Part model, mm, in its own coordinate system. Round coordinates to 2 decimals unless told otherwise and drop trailing zeros. Order: outer loops, then holes, each group sorted by start corner. A loop starts at its lowest first (then second) coordinate and runs counter-clockwise, first axis right, second up. Notation, with made-up numbers: (41, 45.5) -> (96, 45.5) arc R21 cw to (96, 58.5) -> close; hole circle Ø2 at (-27, 53). An arc over 180 degrees is marked (long way). Answer as a JSON object with one key per item and string values. Group by question number.
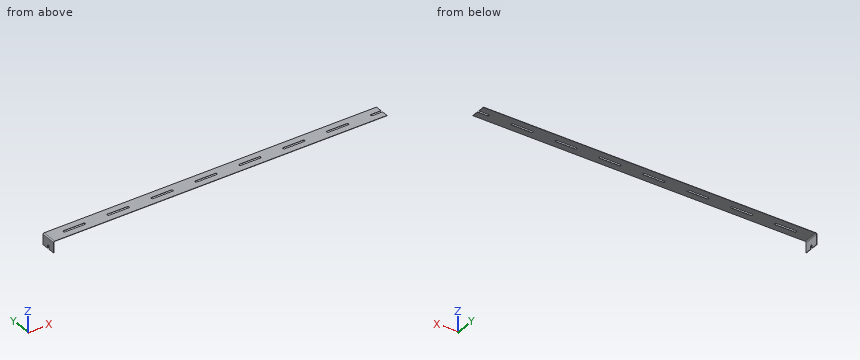
```python
from build123d import *

# Parameters (mm, degrees)
F0_W     = 3
F0_H     = 3
F1_DEPTH = 0.15
F2_DEPTH = 1.9
F3_W     = 0.15
F3_H     = 7
F4_DEPTH = 5
F6_DEPTH = 25
F7_R     = 0.5


with BuildPart() as f1:
    # F0 (on Top) → F1 (new body)
    with BuildSketch(Plane.XY):
        with Locations((72.2, 2)):
            Rectangle(F0_W, F0_H)
        with BuildLine():
            Line((10.1, -0.5), (10.1, -3.5))
            Line((10.1, -3.5), (20.2, -3.5))
            Line((20.2, -3.5), (30.3, -3.5))
            Line((30.3, -3.5), (30.3, -0.5))
            Line((30.3, -0.5), (25.7, -0.5))
            ThreePointArc((25.7, -0.5), (25.4171572875, -0.3828427125), (25.3, -0.1))
            Line((25.3, -0.1), (25.3, 0.1))
            ThreePointArc((25.3, 0.1), (25.4171572875, 0.3828427125), (25.7, 0.5))
            Line((25.7, 0.5), (30.3, 0.5))
            Line((30.3, 0.5), (30.3, 3.5))
            Line((30.3, 3.5), (20.2, 3.5))
            Line((20.2, 3.5), (10.1, 3.5))
            Line((10.1, 3.5), (10.1, 0.5))
            Line((10.1, 0.5), (14.7, 0.5))
            ThreePointArc((14.7, 0.5), (14.9828427125, 0.3828427125), (15.1, 0.1))
            Line((15.1, 0.1), (15.1, -0.1))
            ThreePointArc((15.1, -0.1), (14.9828427125, -0.3828427125), (14.7, -0.5))
            Line((14.7, -0.5), (10.1, -0.5))
        make_face()
        with BuildLine():
            Line((30.3, -0.5), (30.3, -3.5))
            Line((30.3, -3.5), (40.4, -3.5))
            Line((40.4, -3.5), (50.5, -3.5))
            Line((50.5, -3.5), (50.5, -0.5))
            Line((50.5, -0.5), (45.9, -0.5))
            ThreePointArc((45.9, -0.5), (45.6171572875, -0.3828427125), (45.5, -0.1))
            Line((45.5, -0.1), (45.5, 0.1))
            ThreePointArc((45.5, 0.1), (45.6171572875, 0.3828427125), (45.9, 0.5))
            Line((45.9, 0.5), (50.5, 0.5))
            Line((50.5, 0.5), (50.5, 3.5))
            Line((50.5, 3.5), (40.4, 3.5))
            Line((40.4, 3.5), (30.3, 3.5))
            Line((30.3, 3.5), (30.3, 0.5))
            Line((30.3, 0.5), (34.9, 0.5))
            ThreePointArc((34.9, 0.5), (35.1828427125, 0.3828427125), (35.3, 0.1))
            Line((35.3, 0.1), (35.3, -0.1))
            ThreePointArc((35.3, -0.1), (35.1828427125, -0.3828427125), (34.9, -0.5))
            Line((34.9, -0.5), (30.3, -0.5))
        make_face()
        with BuildLine():
            Line((50.5, -0.5), (50.5, -3.5))
            Line((50.5, -3.5), (60.6, -3.5))
            Line((60.6, -3.5), (70.7, -3.5))
            Line((70.7, -3.5), (70.7, -0.5))
            Line((70.7, -0.5), (66.1, -0.5))
            ThreePointArc((66.1, -0.5), (65.8171572875, -0.3828427125), (65.7, -0.1))
            Line((65.7, -0.1), (65.7, 0.1))
            ThreePointArc((65.7, 0.1), (65.8171572875, 0.3828427125), (66.1, 0.5))
            Line((66.1, 0.5), (70.7, 0.5))
            Line((70.7, 0.5), (70.7, 3.5))
            Line((70.7, 3.5), (60.6, 3.5))
            Line((60.6, 3.5), (50.5, 3.5))
            Line((50.5, 3.5), (50.5, 0.5))
            Line((50.5, 0.5), (55.1, 0.5))
            ThreePointArc((55.1, 0.5), (55.3828427125, 0.3828427125), (55.5, 0.1))
            Line((55.5, 0.1), (55.5, -0.1))
            ThreePointArc((55.5, -0.1), (55.3828427125, -0.3828427125), (55.1, -0.5))
            Line((55.1, -0.5), (50.5, -0.5))
        make_face()
        with BuildLine():
            Line((0, 3.5), (0, -3.5))
            Line((0, -3.5), (10.1, -3.5))
            Line((10.1, -3.5), (10.1, -0.5))
            Line((10.1, -0.5), (5.5, -0.5))
            ThreePointArc((5.5, -0.5), (5.2171572875, -0.3828427125), (5.1, -0.1))
            Line((5.1, -0.1), (5.1, 0.1))
            ThreePointArc((5.1, 0.1), (5.2171572875, 0.3828427125), (5.5, 0.5))
            Line((5.5, 0.5), (10.1, 0.5))
            Line((10.1, 0.5), (10.1, 3.5))
            Line((10.1, 3.5), (0, 3.5))
        make_face()
        with Locations((72.2, -2)):
            Rectangle(F0_W, F0_H)
        with BuildLine():
            Line((73.7, -0.5), (73.7, -3.5))
            Line((73.7, -3.5), (80.8, -3.5))
            Line((80.8, -3.5), (90.9, -3.5))
            Line((90.9, -3.5), (90.9, -0.5))
            Line((90.9, -0.5), (86.3, -0.5))
            ThreePointArc((86.3, -0.5), (86.0171572875, -0.3828427125), (85.9, -0.1))
            Line((85.9, -0.1), (85.9, 0.1))
            ThreePointArc((85.9, 0.1), (86.0171572875, 0.3828427125), (86.3, 0.5))
            Line((86.3, 0.5), (90.9, 0.5))
            Line((90.9, 0.5), (90.9, 3.5))
            Line((90.9, 3.5), (80.8, 3.5))
            Line((80.8, 3.5), (73.7, 3.5))
            Line((73.7, 3.5), (73.7, 0.5))
            Line((73.7, 0.5), (75.3, 0.5))
            ThreePointArc((75.3, 0.5), (75.5828427125, 0.3828427125), (75.7, 0.1))
            Line((75.7, 0.1), (75.7, -0.1))
            ThreePointArc((75.7, -0.1), (75.5828427125, -0.3828427125), (75.3, -0.5))
            Line((75.3, -0.5), (73.7, -0.5))
        make_face()
        with BuildLine():
            Line((90.9, -0.5), (90.9, -3.5))
            Line((90.9, -3.5), (101, -3.5))
            Line((101, -3.5), (111.1, -3.5))
            Line((111.1, -3.5), (111.1, -0.5))
            Line((111.1, -0.5), (106.5, -0.5))
            ThreePointArc((106.5, -0.5), (106.2171572875, -0.3828427125), (106.1, -0.1))
            Line((106.1, -0.1), (106.1, 0.1))
            ThreePointArc((106.1, 0.1), (106.2171572875, 0.3828427125), (106.5, 0.5))
            Line((106.5, 0.5), (111.1, 0.5))
            Line((111.1, 0.5), (111.1, 3.5))
            Line((111.1, 3.5), (101, 3.5))
            Line((101, 3.5), (90.9, 3.5))
            Line((90.9, 3.5), (90.9, 0.5))
            Line((90.9, 0.5), (95.5, 0.5))
            ThreePointArc((95.5, 0.5), (95.7828427125, 0.3828427125), (95.9, 0.1))
            Line((95.9, 0.1), (95.9, -0.1))
            ThreePointArc((95.9, -0.1), (95.7828427125, -0.3828427125), (95.5, -0.5))
            Line((95.5, -0.5), (90.9, -0.5))
        make_face()
        with BuildLine():
            Line((111.1, -0.5), (111.1, -3.5))
            Line((111.1, -3.5), (121.2, -3.5))
            Line((121.2, -3.5), (131.3, -3.5))
            Line((131.3, -3.5), (131.3, -0.5))
            Line((131.3, -0.5), (126.7, -0.5))
            ThreePointArc((126.7, -0.5), (126.4171572875, -0.3828427125), (126.3, -0.1))
            Line((126.3, -0.1), (126.3, 0.1))
            ThreePointArc((126.3, 0.1), (126.4171572875, 0.3828427125), (126.7, 0.5))
            Line((126.7, 0.5), (131.3, 0.5))
            Line((131.3, 0.5), (131.3, 3.5))
            Line((131.3, 3.5), (121.2, 3.5))
            Line((121.2, 3.5), (111.1, 3.5))
            Line((111.1, 3.5), (111.1, 0.5))
            Line((111.1, 0.5), (115.7, 0.5))
            ThreePointArc((115.7, 0.5), (115.9828427125, 0.3828427125), (116.1, 0.1))
            Line((116.1, 0.1), (116.1, -0.1))
            ThreePointArc((116.1, -0.1), (115.9828427125, -0.3828427125), (115.7, -0.5))
            Line((115.7, -0.5), (111.1, -0.5))
        make_face()
        with BuildLine():
            Line((131.3, -0.5), (131.3, -3.5))
            Line((131.3, -3.5), (141.4, -3.5))
            Line((141.4, -3.5), (151.5, -3.5))
            Line((151.5, -3.5), (151.5, -0.5))
            Line((151.5, -0.5), (146.9, -0.5))
            ThreePointArc((146.9, -0.5), (146.6171572875, -0.3828427125), (146.5, -0.1))
            Line((146.5, -0.1), (146.5, 0.1))
            ThreePointArc((146.5, 0.1), (146.6171572875, 0.3828427125), (146.9, 0.5))
            Line((146.9, 0.5), (151.5, 0.5))
            Line((151.5, 0.5), (151.5, 3.5))
            Line((151.5, 3.5), (141.4, 3.5))
            Line((141.4, 3.5), (131.3, 3.5))
            Line((131.3, 3.5), (131.3, 0.5))
            Line((131.3, 0.5), (135.9, 0.5))
            ThreePointArc((135.9, 0.5), (136.1828427125, 0.3828427125), (136.3, 0.1))
            Line((136.3, 0.1), (136.3, -0.1))
            ThreePointArc((136.3, -0.1), (136.1828427125, -0.3828427125), (135.9, -0.5))
            Line((135.9, -0.5), (131.3, -0.5))
        make_face()
    extrude(amount=F1_DEPTH)

    # F2 (add): a face of the model
    f2_faces = [f1.faces().sort_by_distance(p)[0] for p in [
        (0, 0, 0.075),
    ]]
    extrude(f2_faces, amount=F2_DEPTH)

    # F3 (on face) → F4 (join)
    with BuildSketch(Plane(origin=(0, 0, 0), x_dir=(1, 0, 0), z_dir=(0, 0, -1))):
        with Locations((-1.825, 0)):
            Rectangle(F3_W, F3_H)
    extrude(amount=F4_DEPTH)

    # F5 (on face) → F6 (cut)
    with BuildSketch(Plane(origin=(-1.9, 0, 0), x_dir=(0, -1, 0), z_dir=(-1, 0, 0))):
        with BuildLine():
            ThreePointArc((0.5, -3.75), (0.3828427125, -3.4671572875), (0.1, -3.35))
            Line((0.1, -3.35), (-0.1, -3.35))
            ThreePointArc((-0.1, -3.35), (-0.3828427125, -3.4671572875), (-0.5, -3.75))
            Line((-0.5, -3.75), (-0.5, -5))
            Line((-0.5, -5), (0.5, -5))
            Line((0.5, -5), (0.5, -3.75))
        make_face()
    extrude(amount=-F6_DEPTH, mode=Mode.SUBTRACT)

    # F7
    f7_edges = [f1.edges().sort_by_distance(p)[0] for p in [
        (-1.9, 0, 0.15),
        (-1.75, 0, 0),
    ]]
    fillet(f7_edges, radius=F7_R)


solid = f1.part
```
Q1. Wall check: line 1 (Z direction, x = 100, y = -1.75); line 2 (X direction, y = -0.5, z = -0.45). Give the ranges that are in metal, low to high. Write a range as [from, to].
Q2. Band-saw the part on C-C (x = 19). List the corners of the cut face in (y, z).
Q3. Band-saw the part on A-A (x = 132). List the corners of the cut face in (y, z).
Q4. Band-saw the part on D-D (z = -2.35). List the corners of the cut face in (x, y).
Q5. Band-saw the part on B-B (y = 2). List the corners of the cut face in (x, z), plus the area to 3 significant figures.
Q6. Drop a flat-ended pin along its axis: pin 1 Ø2 at (x, y) = (20, 0) entering from -Z. Give the stop position or say it passes through.
Completed:
{
 "1": {"line 1": "[0, 0.15]", "line 2": "[-1.9, -1.75]"},
 "2": {"outline": "(-3.5, 0) -> (3.5, 0) -> (3.5, 0.15) -> (-3.5, 0.15) -> close"},
 "3": {"outline": "(-3.5, 0) -> (-0.5, 0) -> (-0.5, 0.15) -> (-3.5, 0.15) -> close; (0.5, 0) -> (3.5, 0) -> (3.5, 0.15) -> (0.5, 0.15) -> close"},
 "4": {"outline": "(-1.9, -3.5) -> (-1.75, -3.5) -> (-1.75, 3.5) -> (-1.9, 3.5) -> close"},
 "5": {"outline": "(-1.9, -5) -> (-1.75, -5) -> (-1.75, -0.5) arc R0.5 cw to (-1.25, 0) -> (151.5, 0) -> (151.5, 0.15) -> (-1.4, 0.15) arc R0.5 ccw to (-1.9, -0.35) -> close", "area": "23.8 mm2"},
 "6": {"pin 1": "z = 0"}
}
